Read the model definition and answer for the solid it produces. Units are mm, in the model's axes. Face numbers are marked on the shaded views. A direction names the side the tool comes from. Coordinates: 2 decimals unless noted, no trailing zeros. Order: outer loops, then holes, each group sorted by start corner. A loop starts at its lowest first (then second) coordinate and runs counter-clockwise, first axis right, second up. Notation, with made-up numbers: (-5, 82) -> (37, 82) arc R9 cw to (37, 96) -> close; hole circle Ø2 at (42, 56.25). An arc over 180 degrees is marked (long way). Return JSON: item names as keys, results as strings. Group by question number.
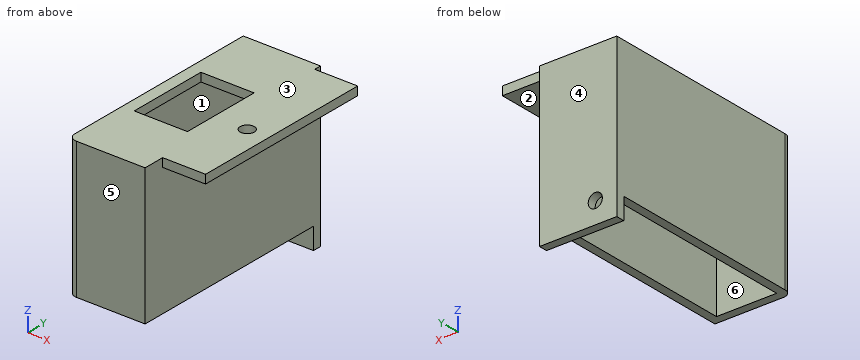
```python
from build123d import *

# Parameters (mm, degrees)
F0_W          = 14
F0_H          = 46
F0_W_2        = 10
F0_H_2        = 43.35
F0_R          = 1.65
F0_W_3        = 12.4
F0_H_3        = 19
F1_DEPTH      = 2
F2_DEPTH      = 30
F4_DEPTH      = 5
F5_R          = 1.65
F6_DEPTH      = 25
F6_DEPTH_BACK = 25


with BuildPart() as f1:
    # F0 (on Top) → F1 (new body)
    with BuildSketch(Plane.XY):
        with BuildLine():
            Line((9, 25), (-9, 25))
            Line((-9, 25), (-9, -23))
            ThreePointArc((-9, -23), (-8.414214, -24.414214), (-7, -25))
            Line((-7, -25), (9, -25))
            Line((9, -25), (9, -20))
            Line((9, -20), (9, 23.35))
            Line((9, 23.35), (9, 25))
        make_face()
        Rectangle(F0_W, F0_H, mode=Mode.SUBTRACT)
        with Locations((14, 1.675)):
            Rectangle(F0_W_2, F0_H_2)
        with Locations((14, -2)):
            Circle(F0_R, mode=Mode.SUBTRACT)
        Rectangle(F0_W, F0_H)
        Rectangle(F0_W_3, F0_H_3, mode=Mode.SUBTRACT)
    extrude(amount=F1_DEPTH)

    # F0 (on Top) → F2 (join)
    with BuildSketch(Plane.XY):
        with BuildLine():
            Line((9, 25), (-9, 25))
            Line((-9, 25), (-9, -23))
            ThreePointArc((-9, -23), (-8.414214, -24.414214), (-7, -25))
            Line((-7, -25), (9, -25))
            Line((9, -25), (9, -20))
            Line((9, -20), (9, 23.35))
            Line((9, 23.35), (9, 25))
        make_face()
        Rectangle(F0_W, F0_H, mode=Mode.SUBTRACT)
    extrude(amount=-F2_DEPTH)

    # F3 (on face) → F4 (join)
    with BuildSketch(Plane(origin=(0, 0, -30), x_dir=(1, 0, 0), z_dir=(0, 0, -1))):
        Polygon((-9, -23), (-9, -25), (9, -25), (9, -23), (7, -23), (-7, -23), align=None)
    extrude(amount=F4_DEPTH)

    # F5 (on face) → F6 (cut, two sides)
    with BuildSketch(Plane(origin=(0, 25, 0), x_dir=(-1, 0, 0), z_dir=(0, 1, 0))) as f6_sk:
        with Locations((4, -30)):
            Circle(F5_R)
    extrude(amount=-F6_DEPTH, mode=Mode.SUBTRACT)
    extrude(f6_sk.sketch, amount=-F6_DEPTH_BACK, mode=Mode.SUBTRACT)


solid = f1.part
```
1. Find section B-B on x = -4. Determine the outline of the cut face in (y, z).
2. Find section D-D on y = 12. Determine the outline of the cut face in (x, z).
3. Straight lines are drawn through the part: L1, parallel to Y at x = 14, z = 1.6; L2, parallel to X at y = 0.5, z = -27.5; L3, parallel to Z at x = -4, y = 23.65. For each, find the intervals that lie inside material, in ascending order.
4. Given pin 1 (15 mm diameter, centred on y = 6, z = -20, fed in from +X); pin 2 (14.5 mm diameter, centred on x = 0, y = -13, fed in from -Z); pin 3 (1.6 mm diameter, centred on x = 13, z = 0.5, fed in from +Y), each flat-ended and moving along its own axis, determine where each tip first touches the part or whether it passes through.
5. For a pull along Y with two mould halves and no side action, classify the marked faces 4, 5 and 6 as released by +Y, released by -Y, zero draft, split by the parting line, or undercut.
6. Find section A-A on x = 14. Determine the outline of the cut face in (y, z), and give its area (3 significant figures).
7. Which of the six approach directions +Z, -Z, +X, -X, +Y, -Y give full straight-line access (tool end or side, diameter ignored) to the marked faces 1, 2 and 3?
8. Find section C-C on z = -10.5. Determine the outline of the cut face in (x, y), and give its area (3 significant figures).
Result:
{
 "1": {"outline": "(-25, -30) -> (-23, -30) -> (-23, 0) -> (-9.5, 0) -> (-9.5, 2) -> (-25, 2) -> close; (9.5, 0) -> (23, 0) -> (23, -28.35) -> (25, -28.35) -> (25, 2) -> (9.5, 2) -> close; (23, -35) -> (25, -35) -> (25, -31.65) -> (23, -31.65) -> close"},
 "2": {"outline": "(-9, -30) -> (-7, -30) -> (-7, 0) -> (7, 0) -> (7, -30) -> (9, -30) -> (9, 0) -> (19, 0) -> (19, 2) -> (-9, 2) -> close"},
 "3": {"L1": "-20 to -3.65, -0.35 to 23.35", "L2": "-9 to -7, 7 to 9", "L3": "-35 to -31.65, -28.35 to 2"},
 "4": {"pin 1": "x = 9", "pin 2": "z = -30", "pin 3": "y = 23.35"},
 "5": {"face 4": "released by +Y", "face 5": "released by -Y", "face 6": "undercut"},
 "6": {"outline": "(-20, 0) -> (-3.65, 0) -> (-3.65, 2) -> (-20, 2) -> close; (-0.35, 0) -> (23.35, 0) -> (23.35, 2) -> (-0.35, 2) -> close", "area": "80.1 mm^2"},
 "7": {"face 1": "-Z", "face 2": "-Z, +X, +Y, -Y", "face 3": "+Z, +X, -X, +Y, -Y"},
 "8": {"outline": "(-9, -23) arc R2 ccw to (-7, -25) -> (9, -25) -> (9, 25) -> (-9, 25) -> close; hole (-7, -23) -> (7, -23) -> (7, 23) -> (-7, 23) -> close", "area": "255 mm^2"}
}
